Geometry check sheet. Reference: drawing and pictorial views, mm from the part's lowest x, y, z. A direction names the side the tool comes from. Round coordinates to 2 decimals unless told otherwise and drop trailing zeros. Write each loop counter-clockwise with the first axis right and the second up, starting at its lowest first coordinate (ties: lowest second). Pieces come first, ordered by that corner, then holes. Notation, with made-up numbers: M 48,32 L 95,32 A11 ccw 95,36 Z; hole C 48.25,69 d2. An arc over 180 degrees is marked long. Put each result on its own line as item: value. Start each with the question number.
(1) Section check C-C on y = 15. Record the cut outline in (x, z) (3 decimals).
(2) Section check A-A on x = 38.1. Record the cut outline in (y, z).
(3) Mould release check, pull along Z, two halves, no side actions. Record for the marked faces 4, 5 and 6: pulls with the +Z half, pulls with the -Z half, needs draft (parallel to the pull), parting line crosses it, or undercut.
(4) Tool access check on the marked faces 1, 2 and 3. Record the directions out of +Z, -Z, +X, -X, +Y, -Y that give a thin tool (end or side, any length) a straight path to the whole face; none if there is none.
(5) Section check B-B on z = 103.5. Record the cut outline in (x, y), then the cut area to 3 significant figures.
(6) Section check D-D on z = 16. Record the cut outline in (x, y), then the cut area to 3 significant figures.
(7) Gauge pin test, flat end, axial feed: pin 1 (15 mm diameter, centred on x = 39, y = 12.5, fed in from +Z). Record the tip position at first contact, or that the pin passes through.
(8) Material ranges on probe 1 along Z at (x, y) = (38.1, 8.75); probe 2 along Y at (x, z) = (65.5, 43), recorded low to high.
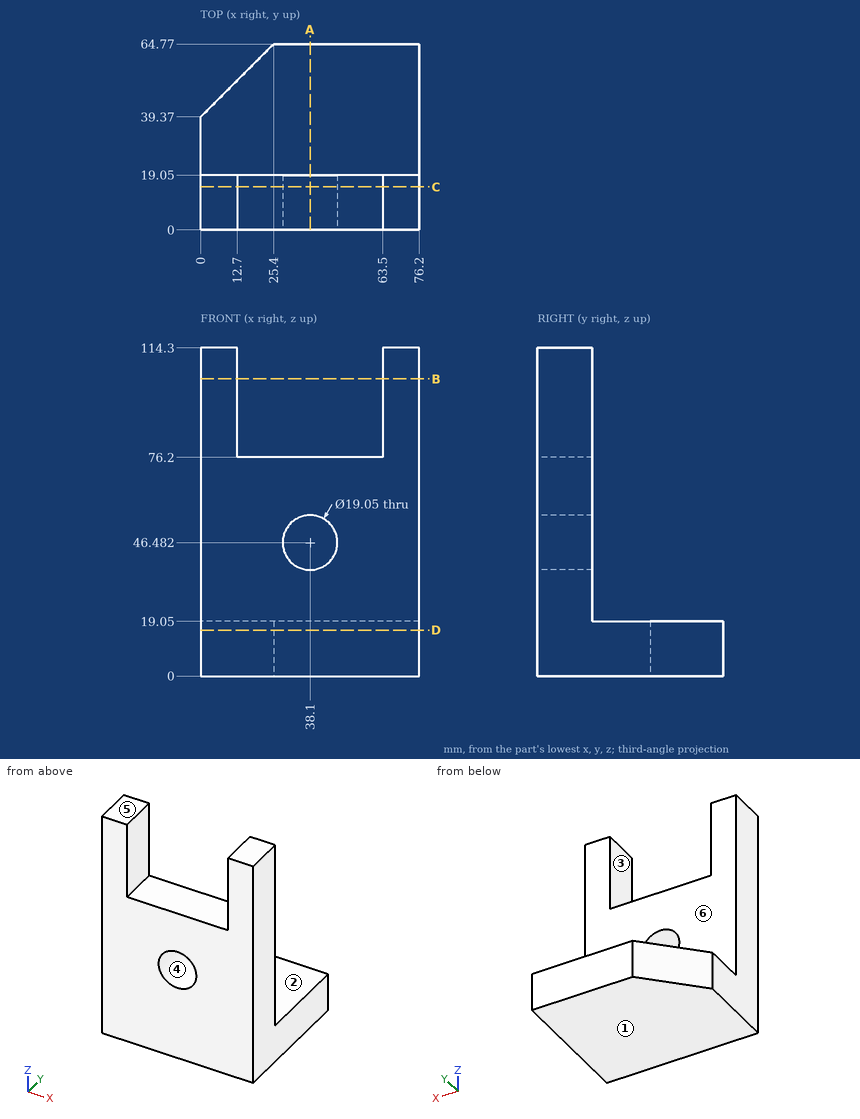
Answers follow:
1. outline: M 0,0 L 76.2,0 L 76.2,114.3 L 63.5,114.3 L 63.5,76.2 L 12.7,76.2 L 12.7,114.3 L 0,114.3 Z; hole C 38.1,46.482 d19.05
2. outline: M 0,0 L 64.77,0 L 64.77,19.05 L 19.05,19.05 L 19.05,36.96 L 0,36.96 Z; M 0,56.01 L 19.05,56.01 L 19.05,76.2 L 0,76.2 Z
3. face 4: undercut
3. face 5: pulls with the +Z half
3. face 6: needs draft
4. face 1: -Z, +X, -X, +Y, -Y
4. face 2: +Z, +X, -X, +Y
4. face 3: +Z, +Y, -Y
5. outline: M 0,0 L 12.7,0 L 12.7,19.05 L 0,19.05 Z; M 63.5,0 L 76.2,0 L 76.2,19.05 L 63.5,19.05 Z
5. area: 484 mm^2
6. outline: M 0,0 L 76.2,0 L 76.2,64.77 L 25.4,64.77 L 0,39.37 Z
6. area: 4,610 mm^2
7. pin 1: stops at z = 76.2
8. probe 1: z = 0 to 36.96, 56.01 to 76.2
8. probe 2: y = 0 to 19.05
